Autodesk Inventor part; units mm, degrees
ref_plane "YZ Plane" through (0, 0, 0) normal (1, 0, 0) x (0, 1, 0)
ref_plane "XZ Plane" through (0, 0, 0) normal (0, 1, 0) x (-1, 0, 0)
ref_plane "XY Plane" through (0, 0, 0) normal (0, 0, 1) x (1, 0, 0)
sketch "Sketch1" plane through (0, 0, 0) normal (0, 0, 1) x (1, 0, 0)
  line L0 (-615, 305) -> (615, 305)
  line L1 (615, 305) -> (615, -305)
  line L2 (615, -305) -> (-615, -305)
  line L3 (-615, -305) -> (-615, 305)
  line L4 (-615, 305) -> (615, -305) construction
  line L5 (615, 305) -> (-615, -305) construction
  point P0 (0, 0)
  dimension "d0" = 610
  dimension "d1" = 1230
extrude "Extrusion1" add sketch "Sketch1" along normal blind 45
sketch "Sketch2" plane through (0, 0, 45) normal (0, 0, 1) x (1, 0, 0)
  line L0 (-600, 290) -> (600, 290)
  line L1 (600, 290) -> (600, -290)
  line L2 (600, -290) -> (-600, -290)
  line L3 (-600, -290) -> (-600, 290)
  line L4 (-600, 290) -> (600, -290) construction
  line L5 (600, 290) -> (-600, -290) construction
  point P0 (0, 0)
  dimension "d4" = 1200
  dimension "d5" = 580
extrude "Extrusion2" cut sketch "Sketch2" against normal blind 20
sketch "Sketch3" plane through (0, 0, 25) normal (0, 0, 1) x (1, 0, 0)
  line L0 (-20, 290) -> (20, 290)
  line L1 (20, 290) -> (20, -290)
  line L2 (20, -290) -> (-20, -290)
  line L3 (-20, -290) -> (-20, 290)
  line L4 (-20, 290) -> (20, -290) construction
  line L5 (20, 290) -> (-20, -290) construction
  line L6 (250, 290) -> (290, 290)
  line L7 (290, 290) -> (290, -290)
  line L8 (290, -290) -> (250, -290)
  line L9 (250, -290) -> (250, 290)
  line L10 (-290, 290) -> (-250, 290)
  line L11 (-250, 290) -> (-250, -290)
  line L12 (-250, -290) -> (-290, -290)
  line L13 (-290, -290) -> (-290, 290)
  line L14 (-600, 290) -> (600, 290)
  line L15 (520, 290) -> (560, 290)
  line L16 (560, 290) -> (560, -290)
  line L17 (560, -290) -> (520, -290)
  line L18 (520, -290) -> (520, 290)
  line L19 (-560, 290) -> (-520, 290)
  line L20 (-520, 290) -> (-520, -290)
  line L21 (-520, -290) -> (-560, -290)
  line L22 (-560, -290) -> (-560, 290)
  point P0 (0, 0)
  point P1 (250, 0)
  point P2 (-250, 0)
  point P3 (520, 0)
  point P4 (290, 0)
  point P5 (-290, 0)
  point P6 (-520, 0)
  dimension "d8" = 580
  dimension "d9" = 40
  dimension "d10" = 250
  dimension "d11" = 40
  dimension "d12" = 40
  dimension "d13" = 250
  dimension "d14" = 40
  dimension "d15" = 230
  dimension "d16" = 580
  dimension "d17" = 40
  dimension "d18" = 230
extrude "Extrusion3" cut sketch "Sketch3" against normal blind 10
sketch "Sketch4" plane through (0, 0, 25) normal (0, 0, 1) x (1, 0, 0)
  line L0 (600, 290) -> (600, -290)
  line L1 (-600, 180) -> (600, 180)
  line L2 (600, 180) -> (600, 140)
  line L3 (600, 140) -> (-600, 140)
  line L4 (-600, 140) -> (-600, 180)
  line L5 (-600, -140) -> (600, -140)
  line L6 (600, -140) -> (600, -180)
  line L7 (600, -180) -> (-600, -180)
  line L8 (-600, -180) -> (-600, -140)
  point P0 (0, 0)
  point P1 (0, 140)
  point P2 (0, -140)
  point P3 (600, -140)
  dimension "d21" = 140
  dimension "d22" = 140
  dimension "d23" = 40
  dimension "d24" = 40
  dimension "d25" = 1200
extrude "Extrusion4" cut sketch "Sketch4" against normal blind 10
sketch "Sketch5" plane through (0, 0, 25) normal (0, 0, 1) x (1, 0, 0)
  circle A0 centre (580, 0) radius 18.5
  point P0 (0, 0)
  dimension "d28" = 37
  dimension "d29" = 580
extrude "Extrusion5" cut sketch "Sketch5" against normal blind 37
equation "\"d30\" = d28"
properties part number "flood tray"
Work out the finished part from the listing and answer in its coordinate system (mm). A direction names the side the tool comes from. Round coordinates to 2 decimals unless told otherwise and drop trailing zeros. Write each loop counter-clockwise with the first axis right and the second up, starting at its lowest first coordinate (ties: lowest second). Pieces come first, ordered by that corner, then holes.
1) A cutting plane is placed at D-D (x = -403). Give the vertices of the cut face in (y, z).
2) A cutting plane is placed at B-B (x = 580). Give the vertices of the cut face in (y, z).
3) Given pin 1 Ø20 at (x, y) = (-580, 254.5) entering from +Z, flat-ended and moving along its own axis, determine where the tip first touches the part or whether it passes through.
4) A cutting plane is placed at C-C (z = 36). Give the vertices of the cut face in (x, y).
5) The mould has two halves that part along X. Classify faces 3 (the flat face through (-615, -4, 22)), 4 (the flat face through (580, 236, 25)), 5 (the flat face through (-3, 295, 45)), 6 (the flat face through (-580, 236, 25)): pulls with the +X half, pulls with the -X half, needs draft (parallel to the pull), parting line crosses it, or undercut.
6) Straight lines are drawn through the part: line 1 (Y direction, x = -226.5, z = 16); line 2 (Y direction, x = 580, z = 17); line 3 (X direction, y = 121.5, z = 15.5). For each, find the intervals that lie inside material, in ascending order.
7) A tool of negligible diameter and unlimited length cuts with its end or side. For faces 1 (the flat face through (-9, 4, 0)), 2 (the flat face through (-580, 2, 25)), from which of +Z, -Z, +X, -X, +Y, -Y can it reach the whole face along a straight path? Write none if from no direction.
Completed:
1. outline: (-305, 0) - (305, 0) - (305, 45) - (290, 45) - (290, 25) - (180, 25) - (180, 15) - (140, 15) - (140, 25) - (-140, 25) - (-140, 15) - (-180, 15) - (-180, 25) - (-290, 25) - (-290, 45) - (-305, 45) - close
2. outline: (-305, 0) - (-18.5, 0) - (-18.5, 25) - (-140, 25) - (-140, 15) - (-180, 15) - (-180, 25) - (-290, 25) - (-290, 45) - (-305, 45) - close; (18.5, 0) - (305, 0) - (305, 45) - (290, 45) - (290, 25) - (180, 25) - (180, 15) - (140, 15) - (140, 25) - (18.5, 25) - close
3. pin 1: stops at z = 25
4. outline: (-615, -305) - (615, -305) - (615, 305) - (-615, 305) - close; hole (-600, -290) - (600, -290) - (600, 290) - (-600, 290) - close
5. face 3: pulls with the -X half
5. face 4: undercut
5. face 5: needs draft
5. face 6: undercut
6. line 1: y = -305 to -180, -140 to 140, 180 to 305
6. line 2: y = -305 to -180, -140 to -18.5, 18.5 to 140, 180 to 305
6. line 3: x = -615 to -560, -520 to -290, -250 to -20, 20 to 250, 290 to 520, 560 to 615
7. face 1: -Z, +X, -X, +Y, -Y
7. face 2: +Z
